Build history of the part. All positions in model axes, mm. Face numbers are marked on the shaded views. A direction names the side the tool comes from. Round coordinates to 2 decimals unless told otherwise and drop trailing zeros. Write each loop counter-clockwise with the first axis right and the second up, starting at its lowest first coordinate (ties: lowest second). Pieces come first, ordered by that corner, then holes. Notation, with made-up numbers: (-7, 70.25) -> (2, 70.25) arc R19 ccw to (2, 88.25) -> close; hole circle Ø1 at (-34, 20). An arc over 180 degrees is marked (long way). Return JSON: item names as keys, results as strings.
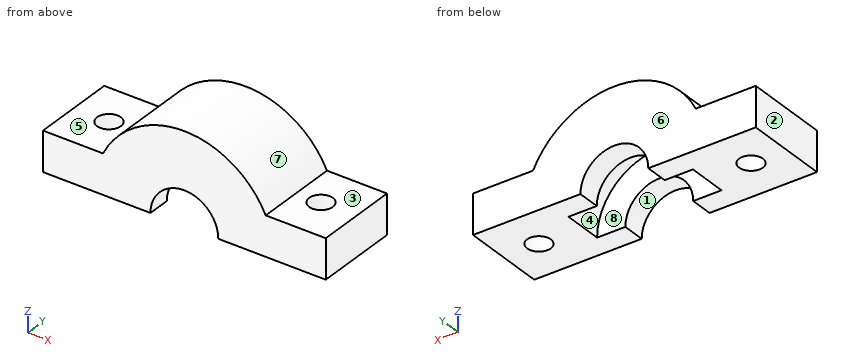
Autodesk Inventor part; units mm, degrees
ref_plane "YZ Plane" through (0, 0, 0) normal (1, 0, 0) x (0, 1, 0)
ref_plane "XZ Plane" through (0, 0, 0) normal (0, 1, 0) x (-1, 0, 0)
ref_plane "XY Plane" through (0, 0, 0) normal (0, 0, 1) x (1, 0, 0)
sketch "Skizze1" plane through (0, 0, 0) normal (0, 0, 1) x (1, 0, 0)
  circle A0 centre (-18.75, 0) radius 2.1
  line L0 (-6.25, 7.5) -> (-6.25, 3.5)
  line L1 (-6.25, 7.5) -> (-25, 7.5)
  line L2 (-25, 7.5) -> (-25, -7.5)
  line L3 (-25, -7.5) -> (-6.25, -7.5)
  line L4 (-6.25, -3.5) -> (-6.25, -7.5)
  line L5 (-11, -3.5) -> (-6.25, -3.5)
  line L6 (-11, 3.5) -> (-11, -3.5)
  line L7 (-6.25, 3.5) -> (-11, 3.5)
  circle A1 centre (18.75, 0) radius 2.1
  line L8 (6.25, 3.5) -> (6.25, 7.5)
  line L9 (11, 3.5) -> (6.25, 3.5)
  line L10 (11, -3.5) -> (11, 3.5)
  line L11 (6.25, -3.5) -> (11, -3.5)
  line L12 (6.25, -7.5) -> (6.25, -3.5)
  line L13 (6.25, -7.5) -> (25, -7.5)
  line L14 (25, -7.5) -> (25, 7.5)
  line L15 (25, 7.5) -> (6.25, 7.5)
  line L16 (-25, 7.5) -> (25, 7.5)
  line L17 (25, 7.5) -> (25, -7.5)
  line L18 (25, -7.5) -> (-25, -7.5)
  line L19 (-25, -7.5) -> (-25, 7.5)
  line L20 (-25, 7.5) -> (25, -7.5) construction
  line L21 (25, 7.5) -> (-25, -7.5) construction
  point P0 (0, 0)
extrude "Extrusion1" add sketch "Skizze1" along normal blind 16
sketch "Skizze2" plane through (-25, -7.5, 0) normal (0, -1, 0) x (1, 0, 0)
  point P0 (25, 0)
ref_plane "Arbeitsebene1" through (-25, 0, 0) normal (0, 1, 0) x (1, 0, 0)
sketch "Skizze3" plane through (-25, 0, 0) normal (0, 1, 0) x (1, 0, 0)
  line L0 (8.35, -16) -> (8.35, 0)
  line L1 (8.35, 0) -> (41.65, 0)
  line L2 (41.65, 0) -> (41.65, -16)
  line L3 (41.65, -16) -> (8.35, -16)
  line L4 (0, -16) -> (0, 0)
  line L5 (0, 0) -> (4.15, 0)
  line L6 (4.15, 0) -> (4.15, -16)
  line L7 (4.15, -16) -> (0, -16)
  line L8 (50, 0) -> (50, -16)
  line L9 (50, -16) -> (45.85, -16)
  line L10 (45.85, -16) -> (45.85, 0)
  line L11 (45.85, 0) -> (50, 0)
  circle A0 centre (25, 0) radius 11
  dimension "d2" = 22
extrude "Extrusion2" cut sketch "Skizze3" along normal mid plane 7 contours A0 L1 | L1 A0
sketch "Skizze4" plane through (-25, 7.5, 0) normal (0, 1, 0) x (1, 0, 0)
  line L0 (50, 0) -> (50, -16)
  line L1 (50, -16) -> (0, -16)
  line L2 (0, -16) -> (0, 0)
  line L3 (0, 0) -> (50, 0)
  line L4 (50, 0) -> (50, -16)
  line L5 (50, -16) -> (0, -16)
  line L6 (0, -16) -> (0, 0)
  line L7 (0, 0) -> (50, 0)
  line L8 (50, 0) -> (50, -16)
  line L9 (50, -16) -> (0, -16)
  line L10 (0, -16) -> (0, 0)
  line L11 (0, 0) -> (50, 0)
  line L12 (50, 0) -> (50, -16)
  line L13 (50, -16) -> (0, -16)
  line L14 (0, -16) -> (0, 0)
  line L15 (0, 0) -> (50, 0)
  line L16 (14, 0) -> (36, 0)
  arc A0 (14, 0) -> (36, 0) centre (25, 0) ccw
  arc A1 (10.6125, -7) -> (39.3875, -7) centre (25, 0) ccw
  line L17 (50, -16) -> (0, -16)
  line L18 (39.3875, -7) -> (50, -7)
  line L19 (10.6125, -7) -> (0, -7)
  dimension "d5" = 7
extrude "Extrusion3" cut sketch "Skizze4" against normal through all contours L0 L1 A1 L18 | L1 L2 L19 A1
sketch "Skizze5" plane through (-25, -7.5, 0) normal (0, -1, 0) x (1, 0, 0)
  circle A0 centre (25, 0) radius 6
  dimension "d8" = 12
extrude "Extrusion4" cut sketch "Skizze5" against normal through all
properties part number "LagerKlemme" material "ABS-Kunststoff"
Q1. Pin check, flat tips, straight feed: pin 1 Ø3 at (x, y) = (-21, -2.5) entering from +Z; pin 2 Ø8.5 at (x, y) = (18, 0.5) entering from +Z; pin 3 Ø4 at (x, y) = (-18.75, 0) entering from -Z; pin 4 Ø8 at (y, z) = (0.5, 12) entering from -X. Stop position of each tip, or through.
Verdict:
{"pin 1": "stops at z = 7", "pin 2": "stops at z = 8.18", "pin 3": "passes through", "pin 4": "stops at x = -13.86"}
Q2. 3-axis set-ups, long thin cutter, end or side, ignore diameter. For the marked faces 1, 2, 3, 4 and 5: which of +Z, -Z, +X, -X, +Y, -Y reach the whole face in a straight line?
Verdict:
{"face 1": "-Z, +Y, -Y", "face 2": "+Z, -Z, -X, +Y, -Y", "face 3": "+Z, +X, +Y, -Y", "face 4": "-Z", "face 5": "+Z, -X, +Y, -Y"}
Q3. Saw through at C-C on z = 10.5. List the corners of the cut face in (x, y).
Verdict:
{"outline": "(-12.07, -7.5) -> (12.07, -7.5) -> (12.07, 7.5) -> (-12.07, 7.5) -> close; hole (-3.28, -3.5) -> (3.28, -3.5) -> (3.28, 3.5) -> (-3.28, 3.5) -> close"}
Q4. Two-plate mould, pull along Y, no slides. Class the marked faces 6, 7 and 8: +Y half, -Y half, draft (parallel to the pull), parting line (faces both ways), or undercut.
Verdict:
{"face 6": "+Y half", "face 7": "draft", "face 8": "undercut"}
Q5. Wall check: L1, parallel to Y at x = -18.75, z = 1.5; L2, parallel to X at y = 0, z = 4.25; L3, parallel to Y at x = -0.5, z = 8.75. Give the ranges that are in metal, low to high.
Verdict:
{"L1": "y = -7.5 to -2.1, 2.1 to 7.5", "L2": "x = -25 to -20.85, -16.65 to -10.15, 10.15 to 16.65, 20.85 to 25", "L3": "y = -7.5 to -3.5, 3.5 to 7.5"}
Q6. Saw through at A-A on x = -18.75. List the corners of the cut face in (y, z).
Verdict:
{"outline": "(-7.5, 0) -> (-2.1, 0) -> (-2.1, 7) -> (-7.5, 7) -> close; (2.1, 0) -> (7.5, 0) -> (7.5, 7) -> (2.1, 7) -> close"}
Q7. Saw through at D-D on x = 0. List the corners of the cut face in (y, z), then the cut area to 3 significant figures.
Verdict:
{"outline": "(-7.5, 6) -> (-3.5, 6) -> (-3.5, 11) -> (3.5, 11) -> (3.5, 6) -> (7.5, 6) -> (7.5, 16) -> (-7.5, 16) -> close", "area": "115 mm²"}
Q8. Saw through at B-B on y = 0. List the corners of the cut face in (x, z).
Verdict:
{"outline": "(-25, 0) -> (-20.85, 0) -> (-20.85, 7) -> (-25, 7) -> close; (-16.65, 0) -> (-11, 0) arc R11 cw to (11, 0) -> (16.65, 0) -> (16.65, 7) -> (14.39, 7) arc R16 ccw to (-14.39, 7) -> (-16.65, 7) -> close; (20.85, 0) -> (25, 0) -> (25, 7) -> (20.85, 7) -> close"}
